Autodesk Inventor part; units mm, degrees
ref_plane "YZ Plane" through (0, 0, 0) normal (1, 0, 0) x (0, 1, 0)
ref_plane "XZ Plane" through (0, 0, 0) normal (0, 1, 0) x (-1, 0, 0)
ref_plane "XY Plane" through (0, 0, 0) normal (0, 0, 1) x (1, 0, 0)
sketch "Sketch1" plane through (0, 0, 0) normal (1, 0, 0) x (0, 1, 0)
  line L0 (0, 0) -> (35, 0)
  line L1 (35, 0) -> (35, 27)
  line L2 (35, 27) -> (0, 27)
  line L3 (0, 27) -> (0, 0)
  line L4 (0, 27) -> (25, 27) construction
  line L5 (25, 27) -> (25, 0) construction
  line L6 (25, 0) -> (0, 0) construction
  line L7 (0, 0) -> (0, 27) construction
  circle A0 centre (12.5, 12.5) radius 6.35
  dimension "d0" = 35
  dimension "d1" = 27
  dimension "d2" = 25
  dimension "d3" = 12.7
extrude "Extrusion1" add sketch "Sketch1" along normal blind 10
sketch "Sketch2" plane through (10, 0, 0) normal (1, 0, 0) x (0, 0, -1)
  line L0 (0, 35) -> (-27, 35)
  line L1 (0, 0) -> (0, 35)
  line L2 (-27, 35) -> (0, 35)
  line L3 (0, 35) -> (0, 25)
  line L4 (0, 25) -> (-27, 25)
  line L5 (-27, 25) -> (-27, 35)
  dimension "d6" = 10
extrude "Extrusion2" add sketch "Sketch2" along normal blind 10
sketch "Sketch3" plane through (10, 0, 0) normal (1, 0, 0) x (0, 0, -1)
  point P0 (0, 0)
sketch "Sketch4" plane through (0, 0, 0) normal (0, 0, -1) x (-1, 0, 0)
  point P0 (0, 0)
sketch "Sketch5" plane through (10, 0, 0) normal (1, 0, 0) x (0, 0, -1)
  point P0 (0, 0)
sketch "Sketch6" plane through (10, 0, 0) normal (1, 0, 0) x (0, 0, -1)
  line L0 (-27, 25) -> (-27, 0)
  line L1 (-27, 0) -> (-22, 0)
  line L2 (-22, 0) -> (-22, 11)
  line L3 (-22, 11) -> (-27, 11)
  line L4 (-27, 11) -> (-27, 0)
  line L5 (-22, 14) -> (-27, 14)
  line L6 (-27, 14) -> (-27, 19)
  line L7 (-27, 19) -> (-22, 19)
  line L8 (-22, 19) -> (-22, 14)
  point P0 (0, 0)
  dimension "d9" = 5
  dimension "d10" = 11
  dimension "d11" = 5
extrude "Extrusion3" add sketch "Sketch6" along normal blind 150
sketch "Sketch7" plane through (10, 19, 27) normal (0, 1, 0) x (1, 0, 0)
  line L0 (-10, 0) -> (10, 0)
  line L1 (0, 5) -> (150, 5)
  line L2 (0, 0) -> (10, 0)
  line L3 (10, 0) -> (10, 5)
  line L4 (10, 5) -> (0, 5)
  line L5 (0, 5) -> (0, 0)
  point P0 (-10, 27)
  dimension "d14" = 10
extrude "Extrusion4" add sketch "Sketch7" along normal blind 7.5
sketch "Sketch8" plane through (160, 0, 0) normal (1, 0, 0) x (0, 0, -1)
  line L0 (-27, 14) -> (-22, 14)
  line L1 (-27, 14) -> (-22, 14)
  line L2 (-22, 25) -> (-22, 14)
  line L3 (-22, 14) -> (-22, 25)
  line L4 (-22, 25) -> (0, 25)
  line L5 (-22, 25) -> (0, 25)
  line L6 (0, 25) -> (0, 35)
  line L7 (0, 25) -> (0, 35)
  line L8 (0, 35) -> (-27, 35)
  line L9 (-27, 35) -> (-27, 14)
  line L10 (-22, 11) -> (-22, 0)
  line L11 (-27, 0) -> (-22, 0)
  line L12 (-22, 0) -> (-22, 11)
  line L13 (-22, 11) -> (-27, 11)
  line L14 (-27, 11) -> (-27, 0)
  point P0 (0, 0)
  dimension "d9" = 5
  dimension "d10" = 11
  dimension "d11" = 5
extrude "Extrusion5" add sketch "Sketch8" along normal blind 10
sketch "Sketch9" plane through (170, 0, 0) normal (1, 0, 0) x (0, 0, -1)
  line L0 (0, 35) -> (-27, 35)
  line L1 (-27, 35) -> (0, 35)
  line L2 (0, 35) -> (0, 0)
  line L3 (0, 0) -> (-27, 0)
  line L4 (-27, 0) -> (-27, 35)
  circle A0 centre (-12.5, 12.5) radius 6.35
  circle A1 centre (-12.5, 12.5) radius 6.35
extrude "Extrusion6" add sketch "Sketch9" along normal blind 10
fillet "Fillet1" radius 2 2 edges at (90, 11, 22) (90, 14, 22)
sketch "Sketch10" plane through (20, 0, 0) normal (1, 0, 0) x (0, 0, -1)
  line L0 (0, 35) -> (-27, 35)
  line L1 (-13.5, 35) -> (-20.5, 35)
  line L2 (-20.5, 35) -> (-6.5, 35)
  line L3 (-20.5, 35) -> (-6.5, 35)
  line L4 (-6.5, 35) -> (-6.5, 32)
  line L5 (-6.5, 32) -> (-20.5, 32)
  line L6 (-20.5, 32) -> (-20.5, 35)
  point P0 (0, 0)
  dimension "d22" = 7
  dimension "d23" = 14
  dimension "d24" = 3
extrude "Extrusion7" add sketch "Sketch10" along normal blind 140
sketch "Sketch11" plane through (0, 35, 27) normal (0, 1, 0) x (1, 0, 0)
  point P0 (0, 27)
sketch "Sketch12" plane through (160, 25, 0) normal (0, 0, -1) x (-1, 0, 0)
  line L0 (-4, 3.5) -> (-16, 3.5)
  line L1 (-16, 3.5) -> (-16, 6.5)
  line L2 (-16, 6.5) -> (-4, 6.5)
  line L3 (-4, 6.5) -> (-4, 3.5)
  line L4 (-4, 3.5) -> (-16, 6.5) construction
  line L5 (-16, 3.5) -> (-4, 6.5) construction
  line L6 (156, 6.5) -> (144, 6.5)
  line L7 (144, 6.5) -> (144, 3.5)
  line L8 (144, 3.5) -> (156, 3.5)
  line L9 (156, 3.5) -> (156, 6.5)
  line L10 (156, 6.5) -> (144, 3.5) construction
  line L11 (144, 6.5) -> (156, 3.5) construction
  point P0 (160, -25)
  point P1 (-10, 5)
  point P2 (150, 5)
  dimension "d27" = 12
  dimension "d28" = 3
  dimension "d29" = 12
  dimension "d30" = 3
extrude "Extrusion8" cut sketch "Sketch12" against normal blind 23.5
sketch "Sketch13" plane through (0, 0, 0) normal (-1, 0, 0) x (0, 0, 1)
  circle A0 centre (12.5, 12.5) radius 6.35 construction
  circle A1 centre (12.5, 12.5) radius 20.6375 construction
  point P0 (0, 0)
  dimension "d33" = 41.275
sketch "Sketch14" plane through (170, 0, 0) normal (-1, 0, 0) x (0, 0, 1)
  circle A0 centre (12.5, 12.5) radius 6.35
  circle A1 centre (12.5, 12.5) radius 6.35
  circle A2 centre (12.5, 12.5) radius 3.5
  point P0 (0, 0)
  dimension "d34" = 7
extrude "Extrusion9" add sketch "Sketch14" against normal blind 4.5
sketch "Sketch15" plane through (10, 0, 0) normal (1, 0, 0) x (0, 0, -1)
  circle A0 centre (-12.5, 12.5) radius 3.5
  circle A1 centre (-12.5, 12.5) radius 6.35
  circle A2 centre (-12.5, 12.5) radius 3.5
  point P0 (0, 0)
  dimension "d37" = 7
extrude "Extrusion10" add sketch "Sketch15" against normal blind 4.5
sketch "Sketch16" plane through (0, 35, 27) normal (0, 1, 0) x (1, 0, 0)
  point P0 (0, 27)
sketch "Sketch17" plane through (20, 19, 27) normal (0, 1, 0) x (1, 0, 0)
  line L0 (-10, 0) -> (150, 0)
  circle A0 centre (70, -3.175) radius 3.175
  line L1 (66.825, 0) -> (73.175, 0)
  line L2 (73.175, 0) -> (73.175, -3.175)
  line L3 (73.175, -3.175) -> (66.825, -3.175)
  line L4 (66.825, -3.175) -> (66.825, 0)
  point P0 (-20, 27)
  point P1 (70, 0)
  point P2 (66.825, -3.175)
  point P3 (73.175, 0)
extrude "Extrusion11" add sketch "Sketch17" against normal blind 19 contours L0 A0 L4 | L0 L2 A0
sketch "Sketch18" plane through (0, 0, 0) normal (-1, 0, 0) x (0, 0, 1)
  point P0 (0, 0)
sketch "Sketch19" plane through (160, 19, 27) normal (0, 0, 1) x (1, 0, 0)
  line L0 (-150, -8) -> (10, -8)
  line L1 (-74.7441, -5.023) -> (-65.8367, -5.023)
  line L2 (-65.8367, -5.023) -> (-65.8367, -8)
  line L3 (-65.8367, -8) -> (-74.7441, -8)
  line L4 (-74.7441, -8) -> (-74.7441, -5.023)
  line L5 (-150, -19) -> (10, -19)
  line L6 (-74.2056, -19) -> (-65.8367, -19)
  line L7 (-65.8367, -19) -> (-65.8367, -17)
  line L8 (-65.8367, -17) -> (-74.2056, -17)
  line L9 (-74.2056, -17) -> (-74.2056, -19)
  point P0 (-160, -19)
  dimension "d42" = 2
extrude "Extrusion12" cut sketch "Sketch19" along normal blind 19
sketch "Sketch20" plane through (0, 35, 27) normal (0, 1, 0) x (1, 0, 0)
  line L0 (0, 0) -> (0, 27)
  line L1 (20, 20.5) -> (160, 20.5)
  line L2 (0, 27) -> (20, 27)
  line L3 (20, 27) -> (20, 20.5)
  line L4 (20, 20.5) -> (0, 20.5)
  line L5 (0, 20.5) -> (0, 27)
extrude "Extrusion13" add sketch "Sketch20" along normal blind 15
sketch "Sketch21" plane through (0, 35, 6.5) normal (0, 0, 1) x (1, 0, 0)
  line L0 (0, 0) -> (20, 0) construction
  line L1 (20, 15) -> (0, 15) construction
  line L2 (0, 0) -> (20, 15) construction
  circle A0 centre (10, 7.5) radius 3.2
  point P0 (0, -35)
  dimension "d47" = 6.4
extrude "Extrusion14" cut sketch "Sketch21" against normal blind 15
sketch "Sketch22" plane through (160, 25, 0) normal (0, 0, -1) x (-1, 0, 0)
  line L0 (-20, 10) -> (-20, -25)
  line L1 (-20, 10) -> (0, 10)
  line L2 (0, 10) -> (0, 25)
  line L3 (0, 25) -> (-20, 25)
  line L4 (-20, 25) -> (-20, 10)
  circle A0 centre (-10, 17.5) radius 3.2
  point P0 (160, -25)
  dimension "d50" = 20
  dimension "d51" = 15
  dimension "d52" = 6.4
extrude "Extrusion15" add sketch "Sketch22" against normal blind 6.5
properties part number "_3DPrint"
The listing builds one solid part. Answer for the finished solid, in the listing's coordinates (mm). A direction names the side the tool comes from. Give positions to 0.01 mm unless a question says otherwise; leave off trailing zeros. Loops run counter-clockwise (first coordinate to the right, second up) from the corner with the lowest first, then second, coordinate; pieces in that order, holes last.
Item 1: Find the intervals of material crossed by line 1 along X through (y, z) = (30, 9); line 2 along Y through (x, z) = (7, 12); line 3 along X through (y, z) = (9, 13), in increasing order.
Derived:
line 1: x = 0 to 4, 16 to 20, 160 to 164, 176 to 180
line 2: y = 0 to 9.04, 15.96 to 28.5, 31.5 to 35
line 3: x = 5.5 to 10, 170 to 174.5
Item 2: A tool of negligible diameter and unlimited length cuts with its end or side. For faces 5 (the flat face through (89, 11, 26)), 6 (the flat face through (164, 30, 12)), 7 (the flat face through (86.825, 7, 29)), from which of +Z, -Z, +X, -X, +Y, -Y can it reach the whole face along a straight path? Write none if from no direction.
Derived:
face 5: +Z, -Z
face 6: -Z
face 7: +Z, -X, +Y, -Y
Item 3: Each of these flat-tipped pins is pushed along its axis until it touches: pin 1 Ø10 at (x, z) = (83.5, 13.5) entering from +Y; pin 2 Ø17.5 at (x, y) = (75.5, 17) entering from +Z; pin 3 Ø1.5 at (x, y) = (105.5, 33) entering from +Z. Where does it stop, or does it pass through?
Derived:
pin 1: stops at y = 35
pin 2: stops at z = 27
pin 3: stops at z = 20.5
Item 4: A cutting plane is placed at C-C (z = 12.5). Give the number of separate pieces and of enclosed holes in the cut face, then the cut area to 3 significant figures.
Derived:
separate pieces: 3
enclosed holes: 2
area: 1,050 mm2
Item 5: Determine the mould class of faces 1 (the cylindrical face through (7.781, 9.083, 13.259)), 2 (the cylindrical face through (90, 7, 27)), 3 (the flat face through (82.9, 0, 22.4)), 4 (the flat face through (89, 14, 25)) for opening direction Y: +Y half, -Y half, draft (parallel to the pull), parting line (faces both ways), or undercut.
Derived:
face 1: undercut
face 2: draft
face 3: -Y half
face 4: undercut
Item 6: A cutting plane is placed at A-A (y = 42.5). Give the vertices of the cut face in (x, z).
Derived:
outline: (0, 0) - (6.8, 0) - (6.8, 6.5) - (0, 6.5) - close; (13.2, 0) - (20, 0) - (20, 6.5) - (13.2, 6.5) - close; (160, 0) - (166.8, 0) - (166.8, 6.5) - (160, 6.5) - close; (173.2, 0) - (180, 0) - (180, 6.5) - (173.2, 6.5) - close
Item 7: A cutting plane is placed at B-B (x = 23). Give the vertices of the cut face in (y, z), then the cut area to 3 significant figures.
Derived:
outline: (0, 22) - (9, 22) arc R2 ccw to (11, 24) - (11, 27) - (0, 27) - close; (14, 24) arc R2 ccw to (16, 22) - (19, 22) - (19, 27) - (14, 27) - close; (32, 6.5) - (35, 6.5) - (35, 20.5) - (32, 20.5) - close
area: 120 mm2
